The listing builds one solid part. Answer for the finished solid, in the listing's coordinates (mm). Face numbers are marked on the shaded views. A direction names the side the tool comes from. Round coordinates to 2 decimals unless told otherwise and drop trailing zeros. Loops run counter-clockwise (first coordinate to the right, second up) from the corner with the lowest first, then second, coordinate; pieces in that order, holes last. Notation, with made-up numbers: (46, 17.5) -> (72, 17.5) arc R26 ccw to (72, 32.5) -> close; hole circle Ø1 at (36, -23.5). An arc over 180 degrees is marked (long way). Use a Markdown table: item, result. Add a question column.
Q1. For a pull along X with two mould halves and no side action, classify the marked faces 1, 2 and 3 as released by +X, released by -X, zero draft, split by the parting line, or undercut.
Q2. Consider line 1 (Z direction, x = -26.15, y = -12.5); line 2 (X direction, y = 18, z = 24.5); line 3 (Z direction, x = -21.5, y = 15.5). Determine where each line is inside the solid, lowest interval first.
Q3. Given pin 1 Ø8 at (x, z) = (-2.5, 3.5) entering from -Y; pin 2 Ø1.5 at (x, z) = (-19.5, 9.5) entering from -Y; pin 3 Ø3.5 at (y, z) = (-12.5, 34.5) entering from +X, each flat-ended and moving along its own axis, determine where each tip first touches the part or whether it passes through.
Q4. Section A-A on y = -12.5 is taken. Give the vertices of the cut face in (x, z).
Q5. Section C-C on z = 29 is taken. Give the vertices of the cut face in (x, y).
Q6. Which of the six approach directions +Z, -Z, +X, -X, +Y, -Y give full straight-line access (tool end or side, diameter ignored) to the marked faces 4 and 5?
Q7. Section D-D on y = 17.5 is taken. Give the vertices of the cut face in (x, z).
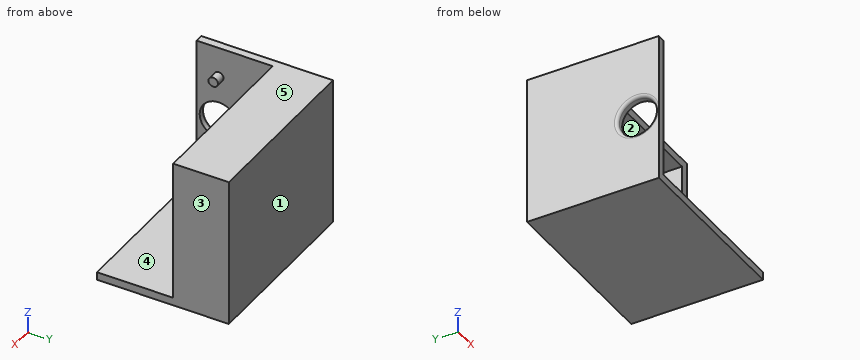
from build123d import *

# Parameters (mm, degrees)
F0_W      = 51
F0_H      = 39
F1_DEPTH  = 2.5
F2_W      = 51
F2_H      = 42
F2_H_2    = 2.5
F3_DEPTH  = 2.5
F4_W      = 39
F4_H      = 42
F4_R      = 6
F5_DEPTH  = 2.5
F6_R      = 0.99999
F7_W      = 51
F7_H      = 15
F8_DEPTH  = 2.5
F9_W      = 15
F9_H      = 42
F10_DEPTH = 2.5
F11_R     = 1.5
F12_DEPTH = 3
F13_DEPTH = 2.5
F14_DEPTH = 2.5


# Not quite as in the source:
# - a fillet or chamfer is up to 0.001 mm smaller than in the source, because OpenCascade refuses the exact size


with BuildPart() as f1:
    # F0 (on Top) → F1 (new body)
    with BuildSketch(Plane.XY):
        Rectangle(F0_W, F0_H)
    extrude(amount=-F1_DEPTH)

    # F2 (on face) → F3 (join)
    with BuildSketch(Plane(origin=(0, 19.5, 0), x_dir=(-1, 0, 0), z_dir=(0, 1, 0))):
        with Locations((0, 21)):
            Rectangle(F2_W, F2_H)
        with Locations((0, -1.25)):
            Rectangle(F2_W, F2_H_2)
    extrude(amount=F3_DEPTH)

    # F4 (on face) → F5 (join)
    with BuildSketch(Plane(origin=(-25.5, 0, 0), x_dir=(0, -1, 0), z_dir=(-1, 0, 0))):
        with Locations((0, 21)):
            Rectangle(F4_W, F4_H)
        with Locations((12.5, 20.5)):
            Circle(F4_R, mode=Mode.SUBTRACT)
        Polygon((19.5, 0), (-19.5, 0), (-19.5, 42), (-22, 42), (-22, -2.5), (19.5, -2.5), align=None)
    extrude(amount=F5_DEPTH)

    # F6 (radius 1 in the source; OpenCascade refuses exactly that, so slightly less here)
    f6_edges = [f1.edges().sort_by_distance(p)[0] for p in [
        (-28, -6.5, 20.5),
    ]]
    fillet(f6_edges, radius=F6_R)

    # F7 (on face) → F8 (join)
    with BuildSketch(Plane.XY.offset(42)):
        Polygon((-25.5, 4.5), (-25.5, 19.5), (25.5, 19.5), (25.5, 22), (-28, 22), (-28, 4.5), align=None)
        with Locations((0, 12)):
            Rectangle(F7_W, F7_H)
    extrude(amount=F8_DEPTH)

    # F9 (on face) → F10 (join)
    with BuildSketch(Plane.YZ.offset(25.5)):
        with Locations((12, 21)):
            Rectangle(F9_W, F9_H)
        Polygon((4.5, 44.5), (4.5, 42), (19.5, 42), (19.5, 0), (4.5, 0), (4.5, -2.5), (22, -2.5), (22, 44.5), align=None)
    extrude(amount=F10_DEPTH)

    # F11 (on face) → F12 (join)
    with BuildSketch(Plane.YZ.offset(-25.5)):
        with Locations((-12.5, 35)):
            Circle(F11_R)
    extrude(amount=F12_DEPTH)

    # F13 (add): a face of the model
    f13_faces = [f1.faces().sort_by_distance(p)[0] for p in [
        (25.5, -7.5, -1.25),
    ]]
    extrude(f13_faces, amount=F13_DEPTH)

    # F14 (add): a face of the model
    f14_faces = [f1.faces().sort_by_distance(p)[0] for p in [
        (-26.75, -7.5, 42),
    ]]
    extrude(f14_faces, amount=F14_DEPTH)


solid = f1.part
Checked values:
| question | item | result |
|---|---|---|
| 1 | face 1 | zero draft |
| 1 | face 2 | undercut |
| 1 | face 3 | released by +X |
| 2 | line 1 | z = -2.5 to 14.5, 26.5 to 44.5 |
| 2 | line 2 | x = -28 to -25.5, 25.5 to 28 |
| 2 | line 3 | z = -2.5 to 0, 42 to 44.5 |
| 3 | pin 1 | stops at y = -19.5 |
| 3 | pin 2 | stops at y = 19.5 |
| 3 | pin 3 | stops at x = -22.5 |
| 4 | outline | (-28, -2.5) -> (28, -2.5) -> (28, 0) -> (-25.5, 0) -> (-25.5, 14.5) -> (-27, 14.5) arc R1 ccw to (-28, 13.5) -> close; (-28, 27.5) arc R1 ccw to (-27, 26.5) -> (-25.5, 26.5) -> (-25.5, 33.5) -> (-22.5, 33.5) -> (-22.5, 36.5) -> (-25.5, 36.5) -> (-25.5, 44.5) -> (-28, 44.5) -> close |
| 5 | outline | (-28, -19.5) -> (-25.5, -19.5) -> (-25.5, 19.5) -> (25.5, 19.5) -> (25.5, 4.5) -> (28, 4.5) -> (28, 22) -> (-28, 22) -> close |
| 6 | face 4 | -Y |
| 6 | face 5 | +Z, +X, -X, +Y, -Y |
| 7 | outline | (-28, -2.5) -> (28, -2.5) -> (28, 44.5) -> (-28, 44.5) -> close; hole (-25.5, 0) -> (25.5, 0) -> (25.5, 42) -> (-25.5, 42) -> close |
